```python
from build123d import *

# Parameters (mm, degrees)
SKETCH_1_R          = 10
EXTRUDE_1_DEPTH     = 8
SKETCH_2_R          = 4.15
CUT_EXTRUDE_1_DEPTH = 5
SKETCH_3_R          = 11.188676277
SKETCH_3_R_2        = 6
CUT_EXTRUDE_2_DEPTH = 5
FILLET_1_R          = 0.5
FILLET_2_R          = 2
SKETCH_4_R          = 3
CUT_EXTRUDE_3_DEPTH = 16


with BuildPart() as part:
    # 草图1 → 凸台-拉伸1 (new body)
    with BuildSketch(Plane.XY):
        Circle(SKETCH_1_R)
    extrude(amount=EXTRUDE_1_DEPTH)

    # 草图2 → 切除-拉伸1 (cut)
    with BuildSketch(Plane(origin=(0, 0, 0), x_dir=(-1, 0, 0), z_dir=(0, 0, -1))):
        Circle(SKETCH_2_R)
    extrude(amount=-CUT_EXTRUDE_1_DEPTH, mode=Mode.SUBTRACT)

    # 草图3 → 切除-拉伸2 (cut)
    with BuildSketch(Plane(origin=(0, 0, 0), x_dir=(-1, 0, 0), z_dir=(0, 0, -1))):
        Circle(SKETCH_3_R)
        Circle(SKETCH_3_R_2, mode=Mode.SUBTRACT)
    extrude(amount=-CUT_EXTRUDE_2_DEPTH, mode=Mode.SUBTRACT)

    # 圆角1
    fillet_1_edges = [part.edges().sort_by_distance(p)[0] for p in [
        (4.15, 0, 0),
    ]]
    fillet(fillet_1_edges, radius=FILLET_1_R)

    # 圆角2
    # the kernel refuses this fillet: 2 mm, written as the material it takes off along each edge
    with BuildSketch(Plane(origin=(0, 0, 5), x_dir=(1, 0, 0), z_dir=(0, 1, 0))) as fillet_2_piece_1:
        with BuildLine():
            CenterArc((10 - FILLET_2_R, -FILLET_2_R), FILLET_2_R, 0, 90)
            Line((10, -FILLET_2_R), (10, 0))
            Line((10, 0), (10 - FILLET_2_R, 0))
        make_face()
    revolve(axis=Axis((0, 0, 5), (0, 0, -1)), mode=Mode.SUBTRACT)
    with BuildSketch(Plane(origin=(0, 0, 0), x_dir=(-1, 0, 0), z_dir=(0, -1, 0))) as fillet_2_piece_2:
        with BuildLine():
            CenterArc((4, -1.891428032), FILLET_2_R, 0, 71.034425011)
            Line((6, -1.891428032), (6, 0))
            Line((6, 0), (4.65, 0))
        make_face()
    revolve(axis=Axis((0, 0, 0), (0, 0, -1)), mode=Mode.SUBTRACT)

    # 草图4 → 切除-拉伸3 (cut, through all)
    with BuildSketch(Plane(origin=(0, 0, 5), x_dir=(-1, 0, 0), z_dir=(0, 0, -1))):
        Circle(SKETCH_4_R)
    extrude(amount=-CUT_EXTRUDE_3_DEPTH, mode=Mode.SUBTRACT)


solid = part.part
```
Can you work these out from the model? Positions are in its coordinate system, mm. A direction names the side the tool comes from. Give positions to 0.01 mm unless a question says otherwise; leave off trailing zeros. Order: outer loops, then holes, each group sorted by start corner. A loop starts at its lowest first (then second) coordinate and runs counter-clockwise, first axis right, second up. Notation, with made-up numbers: M 61.25,60.5 L 68.25,60.5 A23 ccw 68.25,72.5 Z; hole C 56.25,37.25 d1. An arc over 180 degrees is marked long. Write item = value, one per line. Start each with the question number.
Q1. For faces 1 (the flat face through (-1, -3, 5)), 2 (the flat face through (2.1, 2.4, 8)), which set-ups out of +Z, -Z, +X, -X, +Y, -Y let a thin tool reach every point of the face, with its end or its side?
Q2. We'd pull the mould along X, two halves only. Please class faces 3 (the cylindrical face through (-2.17, -9.76, 7.49)), 4 (the flat face through (2, 6, 5)), 5 (the cylindrical face through (0.9, -4.05, 2.72)): pulls with the +X half, pulls with the -X half, needs draft (parallel to the pull), parting line crosses it, or undercut.
Q3. Suppose I cut it at A-A (x = 0). Write out the boundary of the cut face in (y, z), plus the area to 3 significant figures.
Q4. Suppose I cut it at C-C (z = 3.25). Write out the boundary of the cut face in (x, y), plus the area to 3 significant figures.
Q5. Will these pins go through, and if not, where does the flat tip stop? pin 1 Ø2 at (x, z) = (1, 1) entering from +Y; pin 2 Ø6.5 at (x, y) = (0, 0) entering from -Z; pin 3 Ø2 at (y, z) = (4, 2.5) entering from -X.
Q6. I need wall thicknesses on probe 1 along Y at (x, z) = (0, 3.6); probe 2 along Z at (x, y) = (-5.5, -3); probe 3 along Y at (x, z) = (0, 1.4). Which ranges of each line are inside material? Lowest first, please. Write a range as [from, to].
Check result:
q1.face_1 = -Z
q1.face_2 = +Z, +X, -X, +Y, -Y
q2.face_3 = parting line crosses it
q2.face_4 = needs draft
q2.face_5 = undercut
q3.outline = M -10,7 A2 ccw -8,5 L -6,5 L -6,1.89 A2 ccw -4.65,0 A0.5 ccw -4.15,0.5 L -4.15,5 L -3,5 L -3,8 L -10,8 Z; M 3,5 L 4.15,5 L 4.15,0.5 A0.5 ccw 4.65,0 A2 ccw 6,1.89 L 6,5 L 8,5 A2 ccw 10,7 L 10,8 L 3,8 Z
q3.area = 57.3 mm2
q4.outline = C 0,0 d12; hole C 0,0 d8.3
q4.area = 59.0 mm2
q5.pin_1 = 5.99
q5.pin_2 = 5
q5.pin_3 = -5.2
q6.probe_1 = [-6, -4.15], [4.15, 6]
q6.probe_2 = [5, 8]
q6.probe_3 = [-5.94, -4.15], [4.15, 5.94]
